The drawing under review shows one solid part. Ordinate dimensions are in mm from its lowest x, y, z. A direction names the side the tool comes from. Coordinates: 2 decimals unless noted, no trailing zeros. Loops run counter-clockwise (first coordinate to the right, second up) from the corner with the lowest first, then second, coordinate; pieces in that order, holes last. Notation, with made-up numbers: M 87.25,80 L 98.25,80 A19 ccw 98.25,87 Z; hole C 55,2.25 d4. An arc over 180 degrees is marked long. Put each result on its own line as item: value.
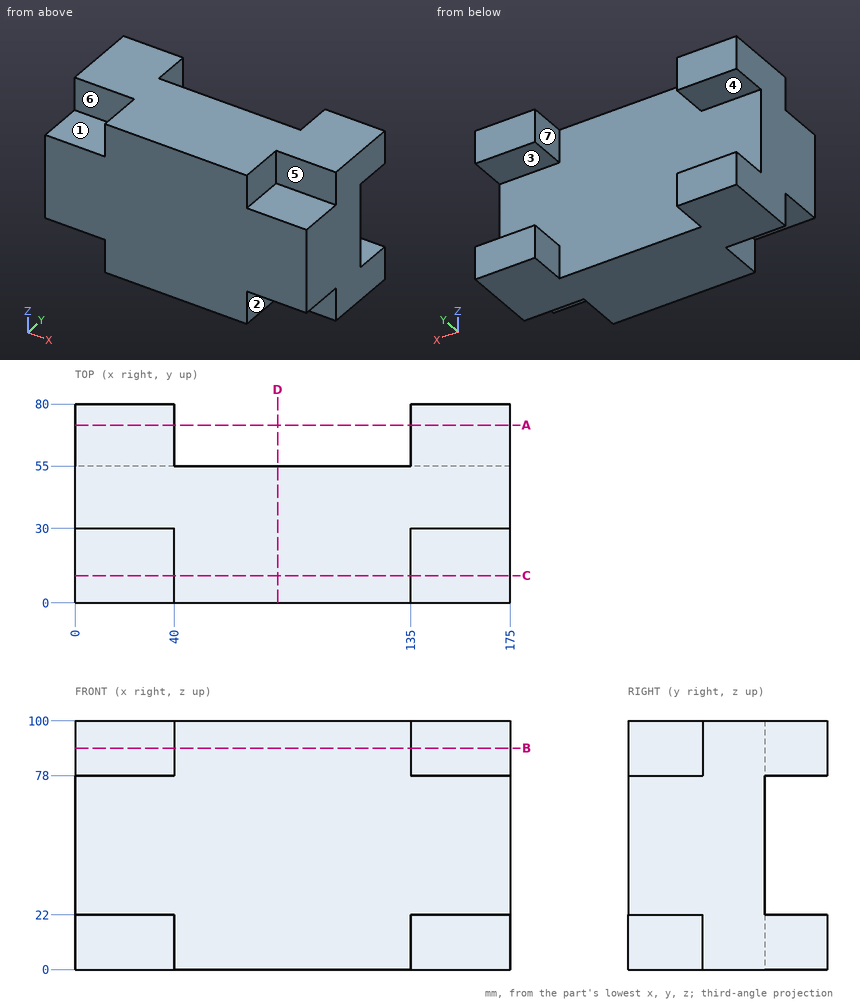
(1) Wall thickness on line 1 along Z through (x, y) = (20.5, 65.5); line 2 along X through (y, z) = (73, 94.5); line 3 along Z through (x, y) = (11.5, 5.5): over which ranges is each line inside the solid? List them lowest first. Write a range as [from, to].
Determined:
line 1: z = [0, 22], [78, 100]
line 2: x = [0, 40], [135, 175]
line 3: z = [22, 78]
(2) Add section D-D (x = 81.5). Write out the cut boundary in (y, z), plus the area to 3 significant figures.
Determined:
outline: M 0,0 L 55,0 L 55,100 L 0,100 Z
area: 5,500 mm^2
(3) Draft analysis for pull direction Z (two halves, no side actions). For the marked faces 1, 2, 3 and 4, state which applies: +Z half, -Z half, draft (parallel to the pull), parting line (faces both ways), or undercut.
Determined:
face 1: +Z half
face 2: draft
face 3: undercut
face 4: undercut
(4) Add section A-A (y = 71.5). Write out the cut boundary in (x, z).
Determined:
outline: M 0,0 L 40,0 L 40,22 L 0,22 Z; M 0,78 L 40,78 L 40,100 L 0,100 Z; M 135,0 L 175,0 L 175,22 L 135,22 Z; M 135,78 L 175,78 L 175,100 L 135,100 Z
(5) Add section C-C (y = 11). Write out the cut boundary in (x, z), plus the area to 3 significant figures.
Determined:
outline: M 0,22 L 40,22 L 40,0 L 135,0 L 135,22 L 175,22 L 175,78 L 135,78 L 135,100 L 40,100 L 40,78 L 0,78 Z
area: 14,000 mm^2
(6) Add section B-B (z = 89). Write out the cut boundary in (x, y), plus the area to 4 significant figures.
Determined:
outline: M 0,30 L 40,30 L 40,0 L 135,0 L 135,30 L 175,30 L 175,80 L 135,80 L 135,55 L 40,55 L 40,80 L 0,80 Z
area: 9,225 mm^2
(7) Tool access review of the marked faces 5, 6 and 7: name each direction out of +Z, -Z, +X, -X, +Y, -Y from which nothing blocks a thin tool from reaching the whole face with its end or side.
Determined:
face 5: +Z, +X, -Y
face 6: +Z, -X, -Y
face 7: +Z, -Z, +Y
(8) For pin 1 (6.5 mm diameter, centred on x = 13.5, z = 12.5, fed in from -Y); pin 2 (9 mm diameter, centred on x = 161, y = 9.5, fed in from +Z); pin 3 (10 mm diameter, centred on x = 43, z = 27, fed in from +Y), all flat-tipped, find the tip position at first contact; note any pin that passes through.
Determined:
pin 1: stops at y = 30
pin 2: stops at z = 78
pin 3: stops at y = 55
